Geometry: final body of the model. Coordinates: model frame, mm. Face numbers are marked on the shaded views. A direction names the side the tool comes from. Give positions to 0.01 mm unless a question says otherwise; leave off trailing zeros. Loops run counter-clockwise (first coordinate to the right, second up) from the corner with the lowest first, then second, coordinate; pieces in that order, holes last.
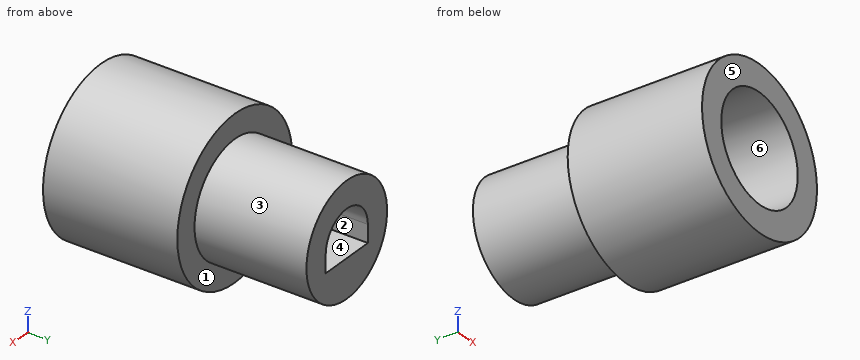
from build123d import *

# Parameters (mm, degrees)
SKETCH1_R           = 7.1625
SKETCH1_R_2         = 4.7625
BOSS_EXTRUDE1_DEPTH = 10
SKETCH2_R           = 7.1625
SKETCH2_R_2         = 4.7625
BOSS_EXTRUDE2_DEPTH = 2
SKETCH3_R           = 5.025
BOSS_EXTRUDE3_DEPTH = 10


with BuildPart() as part:
    # Sketch1 → Boss-Extrude1 (new body)
    with BuildSketch(Plane(origin=(0, 0, 0), x_dir=(1, 0, 0), z_dir=(0, 1, 0))):
        Circle(SKETCH1_R)
        Circle(SKETCH1_R_2, mode=Mode.SUBTRACT)
    extrude(amount=BOSS_EXTRUDE1_DEPTH)

    # Sketch2 → Boss-Extrude2 (add)
    with BuildSketch(Plane(origin=(0, 10, 0), x_dir=(1, 0, 0), z_dir=(0, 1, 0))):
        Circle(SKETCH2_R)
        Circle(SKETCH2_R_2, mode=Mode.SUBTRACT)
        Circle(SKETCH2_R_2)
    extrude(amount=BOSS_EXTRUDE2_DEPTH)

    # Sketch3 → Boss-Extrude3 (add)
    with BuildSketch(Plane(origin=(0, 12, 0), x_dir=(1, 0, 0), z_dir=(0, 1, 0))):
        Circle(SKETCH3_R)
        with BuildLine():
            Line((-2.625, 0), (-2.625, 1.575))
            Line((-2.625, 1.575), (2.625, 1.575))
            Line((2.625, 1.575), (2.625, 0))
            ThreePointArc((2.625, 0), (0, -2.625), (-2.625, 0))
        make_face(mode=Mode.SUBTRACT)
    extrude(amount=BOSS_EXTRUDE3_DEPTH)


solid = part.part
Item 1: Section query D-D on x = 3. Return loops of the section in (y, z), plus the area to 3 significant figures.
Values follow:
outline: (0, -6.5) - (12, -6.5) - (12, -4.03) - (22, -4.03) - (22, 4.03) - (12, 4.03) - (12, 6.5) - (0, 6.5) - (0, 3.7) - (10, 3.7) - (10, -3.7) - (0, -3.7) - close
area: 163 mm2
Item 2: Pin query (flat end, axial travel): pin 1 (0.8 mm diameter, centred on y = 17, z = -1, fed in from +X); pin 2 (1 mm diameter, centred on x = 3, y = 3, fed in from -Z); pin 3 (1.3 mm diameter, centred on x = 0.5, z = 1, fed in from +Y). Return the tip coordinate at first contact, or that it passes through.
Values follow:
pin 1: stops at x = 4.99
pin 2: stops at z = -6.71
pin 3: stops at y = 12
Item 3: Ray query, probe 1 along Z at (x, y) = (0, 6.5); probe 2 along X at (y, z) = (17, 0) (3 decimals); probe 3 along Y at (x, z) = (-0.25, 0.75). Return the intervals inside material, ascending.
Values follow:
probe 1: z = -7.16 to -4.76, 4.76 to 7.16
probe 2: x = -5.025 to -2.625, 2.625 to 5.025
probe 3: y = 10 to 12
Item 4: Draft query along X for the marked faces 1, 2 and 3. Return one class per face: +X half, -X half, draft (parallel to the pull), parting line (faces both ways), or undercut.
Values follow:
face 1: draft
face 2: undercut
face 3: parting line
Item 5: Section query A-A on x = 0. Return loops of the section in (y, z) (1 decimal).
Values follow:
outline: (0, -7.2) - (12, -7.2) - (12, -5) - (22, -5) - (22, -1.6) - (12, -1.6) - (12, 2.6) - (22, 2.6) - (22, 5) - (12, 5) - (12, 7.2) - (0, 7.2) - (0, 4.8) - (10, 4.8) - (10, -4.8) - (0, -4.8) - close
Item 6: Section query C-C on z = -4.25. Return loops of the section in (x, y).
Values follow:
outline: (-5.77, 0) - (-2.15, 0) - (-2.15, 10) - (2.15, 10) - (2.15, 0) - (5.77, 0) - (5.77, 12) - (2.68, 12) - (2.68, 22) - (-2.68, 22) - (-2.68, 12) - (-5.77, 12) - close
Item 7: Section query B-B on y = 17.25. Return loops of the section in (x, z) (3 decimals).
Values follow:
outline: circle Ø10.05 at (0, 0); hole (-2.625, -1.575) - (2.625, -1.575) - (2.625, 0) arc R2.625 ccw to (-2.625, 0) - close
Item 8: Set-up query: the marked faces 4, 5 and 6. Return all of +Z, -Z, +X, -X, +Y, -Y with unobstructed straight access to the full face (end or side cutting, diameter ignored); none if empty.
Values follow:
face 4: +Y
face 5: +Z, -Z, +X, -X, -Y
face 6: -Y
